Verification items for the finished model (mm, model axes). Round coordinates to 2 decimals unless told otherwise and drop trailing zeros. Order: outer loops, then holes, each group sorted by start corner. A loop starts at its lowest first (then second) coordinate and runs counter-clockwise, first axis right, second up. Notation, with made-up numbers: (-40, 63.5) -> (-33, 63.5) arc R20 ccw to (-33, 90.5) -> close; hole circle Ø2 at (81, 82). An arc over 180 degrees is marked (long way). Return JSON: item names as keys, results as strings. Group by question number.
1) Scan lines: L1, parallel to Y at x = -10.92, z = 1.45; L2, parallel to X at y = 10, z = 0.25; L3, parallel to Y at x = -9, z = 0.1. Record each from-to range of solid material in increasing order.
2) Section check D-D on y = 0. Enter the section's corners in (x, z), plus the area to 3 significant figures.
3) Draft check along Y on faces 1 (the cylindrical face through (-9.87, 12.53, 0.99)), 2 (the flat face through (0, 0, 0)), 3 (the flat face through (0, -16.6, 1)). Enter one of: pulls with the +Y half, pulls with the -Y half, needs draft (parallel to the pull), parting line crosses it, or undercut.
4) Section check C-C on x = 5. Enter the section's corners in (y, z), plus the area to 3 significant figures.
5) Section check A-A on x = -10.92. Enter the section's corners in (y, z).
6) Depth check by flat-ended pin: pin 1 (0.5 mm diameter, centred on y = -17, z = 1, fed in from +X). Enter the tip coordinate at first touch or a pass-through.
7) Section check B-B on y = 15.02. Enter the section's corners in (x, z), plus the area to 3 significant figures.
```python
from build123d import *

# Parameters (mm, degrees)
SKETCH_1_W               = 25
SKETCH_1_H               = 33.2
EXTRUDE_1_DEPTH          = 2
FILLET_1_R               = 0.8
CHAMFER_1_SIZE           = 0.2
SKETCH_3_R               = 1.05
CUT_EXTRUDE_2_DEPTH      = 21.876062847
EXTRUDE_2_REACH          = 37.532
CUT_EXTRUDE_3_DEPTH      = 22.148581513
CUT_EXTRUDE_3_DEPTH_BACK = 22.148581513
SKETCH_5_W               = 0.45
SKETCH_5_H               = 9
SKETCH_5_H_2             = 9.2
EXTRUDE_START            = -25
EXTRUDE_3_DEPTH          = 25
CUT_EXTRUDE_4_DEPTH      = 22.503604349
CUT_EXTRUDE_4_DEPTH_BACK = 22.503604349
SKETCH_7_W               = 7
SKETCH_7_H               = 0.45


with BuildPart() as part:
    # 草图1 → 凸台-拉伸1 (new body)
    with BuildSketch(Plane.XY):
        Rectangle(SKETCH_1_W, SKETCH_1_H)
    extrude(amount=EXTRUDE_1_DEPTH)

    # 圆角1
    fillet_1_edges = [part.edges().sort_by_distance(p)[0] for p in [
        (-12.5, 16.6, 1),
        (12.5, 16.6, 1),
        (12.5, -16.6, 1),
        (-12.5, -16.6, 1),
    ]]
    fillet(fillet_1_edges, radius=FILLET_1_R)

    # 倒角1
    chamfer_1_edges = [part.edges().sort_by_distance(p)[0] for p in [
        (12.5, 0, 2),
        (0, -16.6, 2),
        (-12.5, 0, 2),
        (0, 16.6, 2),
        (12.265685425, 16.365685425, 2),
        (-12.265685425, 16.365685425, 2),
        (-12.265685425, -16.365685425, 2),
        (12.265685425, -16.365685425, 2),
    ]]
    chamfer(chamfer_1_edges, length=CHAMFER_1_SIZE)

    # 草图3 → 切除-拉伸2 (cut, through all)
    with BuildSketch(Plane(origin=(0, 0, 0), x_dir=(-1, 0, 0), z_dir=(0, 0, -1))):
        with Locations((10.92, 15.02)):
            Circle(SKETCH_3_R)
        with Locations((8.38, 15.02)):
            Circle(SKETCH_3_R)
        with Locations((5.84, 15.02)):
            Circle(SKETCH_3_R)
        with Locations((8.38, 12.48)):
            Circle(SKETCH_3_R)
        with Locations((5.84, 12.48)):
            Circle(SKETCH_3_R)
        with Locations((8.38, 9.94)):
            Circle(SKETCH_3_R)
        with Locations((5.84, 9.94)):
            Circle(SKETCH_3_R)
        with Locations((8.38, 7.4)):
            Circle(SKETCH_3_R)
        with Locations((5.84, 7.4)):
            Circle(SKETCH_3_R)
        with Locations((10.92, 12.48)):
            Circle(SKETCH_3_R)
        with Locations((10.92, 9.94)):
            Circle(SKETCH_3_R)
        with Locations((10.92, 7.4)):
            Circle(SKETCH_3_R)
    extrude(amount=-CUT_EXTRUDE_2_DEPTH, mode=Mode.SUBTRACT)

    # 凸台-拉伸2: up to this face of the body (flat: up to its plane)
    extrude_2_end = Plane(part.part.faces().sort_by_distance((0, 16.6, 0.9))[0])
    # 草图4 → 凸台-拉伸2 (add, up to the picked face)
    with BuildSketch(Plane.XZ.offset(16.6), mode=Mode.PRIVATE) as extrude_2_sk1:
        Polygon((12.5, 1.45), (12.95, 1), (12.5, 0.55), align=None)
    extrude_2_tool1 = split(extrude(extrude_2_sk1.sketch, amount=-EXTRUDE_2_REACH, mode=Mode.PRIVATE), bisect_by=extrude_2_end, keep=Keep.BOTH, mode=Mode.PRIVATE)
    # 草图4 → 凸台-拉伸2 (add, up to the picked face)
    with BuildSketch(Plane.XZ.offset(16.6), mode=Mode.PRIVATE) as extrude_2_sk2:
        Polygon((-12.5, 1.45), (-12.95, 1), (-12.5, 0.55), align=None)
    extrude_2_tool2 = split(extrude(extrude_2_sk2.sketch, amount=-EXTRUDE_2_REACH, mode=Mode.PRIVATE), bisect_by=extrude_2_end, keep=Keep.BOTH, mode=Mode.PRIVATE)
    add(extrude_2_tool1.solids().sort_by(Axis((12.65, -16.6, 1), (0, 1, 0)))[0])
    add(extrude_2_tool2.solids().sort_by(Axis((-12.65, -16.6, 1), (0, 1, 0)))[0])

    # 草图5 → 切除-拉伸3 (cut, two sides: drawn at the far end of the back side and taken through both)
    with BuildSketch(Plane.XY.offset(2).offset(-CUT_EXTRUDE_3_DEPTH_BACK)):
        with Locations((-12.725, 12.1)):
            Rectangle(SKETCH_5_W, SKETCH_5_H)
        with Locations((-12.725, 0)):
            Rectangle(SKETCH_5_W, SKETCH_5_H_2)
        with Locations((-12.725, -12.1)):
            Rectangle(SKETCH_5_W, SKETCH_5_H)
        with Locations((12.725, -12.1)):
            Rectangle(SKETCH_5_W, SKETCH_5_H)
        with Locations((12.725, 0)):
            Rectangle(SKETCH_5_W, SKETCH_5_H_2)
        with Locations((12.725, 12.1)):
            Rectangle(SKETCH_5_W, SKETCH_5_H)
    extrude(amount=CUT_EXTRUDE_3_DEPTH + CUT_EXTRUDE_3_DEPTH_BACK, mode=Mode.SUBTRACT)

    # 草图6 → 凸台-拉伸3 (add)
    with BuildSketch(Plane(origin=(12.5, 0, 0), x_dir=(0, 0, -1), z_dir=(1, 0, 0)).offset(EXTRUDE_START)):
        Polygon((-1.45, 16.6), (-0.55, 16.6), (-1, 17.05), align=None)
        Polygon((-0.55, -16.6), (-1, -17.05), (-1.45, -16.6), align=None)
    extrude(amount=EXTRUDE_3_DEPTH)

    # 草图7 → 切除-拉伸4 (cut, two sides: drawn at the far end of the back side and taken through both)
    with BuildSketch(Plane.XY.offset(2).offset(-CUT_EXTRUDE_4_DEPTH_BACK)):
        with Locations((-9, 16.825)):
            Rectangle(SKETCH_7_W, SKETCH_7_H)
        with Locations((0, 16.825)):
            Rectangle(SKETCH_7_W, SKETCH_7_H)
        with Locations((9, -16.825)):
            Rectangle(SKETCH_7_W, SKETCH_7_H)
        with Locations((9, 16.825)):
            Rectangle(SKETCH_7_W, SKETCH_7_H)
        with Locations((0, -16.825)):
            Rectangle(SKETCH_7_W, SKETCH_7_H)
        with Locations((-9, -16.825)):
            Rectangle(SKETCH_7_W, SKETCH_7_H)
    extrude(amount=CUT_EXTRUDE_4_DEPTH + CUT_EXTRUDE_4_DEPTH_BACK, mode=Mode.SUBTRACT)


solid = part.part
```
Check result:
{
 "1": {"L1": "-16.6 to 6.35, 8.45 to 8.89, 10.99 to 11.43, 13.53 to 13.97, 16.07 to 16.6", "L2": "-12.5 to -11.97, -9.87 to -9.43, -7.33 to -6.89, -4.79 to 12.5", "L3": "-16.6 to 6.55, 8.25 to 9.09, 10.79 to 11.63, 13.33 to 14.17, 15.87 to 16.6"},
 "2": {"outline": "(-12.5, 0) -> (12.5, 0) -> (12.5, 1.8) -> (12.3, 2) -> (-12.3, 2) -> (-12.5, 1.8) -> close", "area": "50.0 mm^2"},
 "3": {"face 1": "undercut", "face 2": "needs draft", "face 3": "pulls with the -Y half"},
 "4": {"outline": "(-17.05, 1) -> (-16.6, 0.55) -> (-16.6, 0) -> (16.6, 0) -> (16.6, 0.55) -> (17.05, 1) -> (16.6, 1.45) -> (16.6, 1.8) -> (16.4, 2) -> (-16.4, 2) -> (-16.6, 1.8) -> (-16.6, 1.45) -> close", "area": "66.8 mm^2"},
 "5": {"outline": "(-16.6, 0) -> (6.35, 0) -> (6.35, 2) -> (-16.4, 2) -> (-16.6, 1.8) -> close; (8.45, 0) -> (8.89, 0) -> (8.89, 2) -> (8.45, 2) -> close; (10.99, 0) -> (11.43, 0) -> (11.43, 2) -> (10.99, 2) -> close; (13.53, 0) -> (13.97, 0) -> (13.97, 2) -> (13.53, 2) -> close; (16.07, 0) -> (16.6, 0) -> (16.6, 1.8) -> (16.4, 2) -> (16.07, 2) -> close"},
 "6": {"pin 1": "x = 5.5"},
 "7": {"outline": "(-12.5, 0) -> (-11.97, 0) -> (-11.97, 2) -> (-12.3, 2) -> (-12.5, 1.8) -> close; (-9.87, 0) -> (-9.43, 0) -> (-9.43, 2) -> (-9.87, 2) -> close; (-7.33, 0) -> (-6.89, 0) -> (-6.89, 2) -> (-7.33, 2) -> close; (-4.79, 0) -> (12.5, 0) -> (12.5, 1.8) -> (12.3, 2) -> (-4.79, 2) -> close", "area": "37.4 mm^2"}
}
